```python
from build123d import *

# Parameters (mm, degrees)
SKETCH1_W           = 91.44
SKETCH1_H           = 91.44
BOSS_EXTRUDE1_DEPTH = 3.175
SKETCH2_R           = 38.1
BOSS_EXTRUDE2_DEPTH = 2.286
SKETCH3_R           = 1.143
BOSS_EXTRUDE3_DEPTH = 4.572
SKETCH4_R           = 2.667
CUT_EXTRUDE1_DEPTH  = 104.048504199
FILLET1_R           = 2.032
FILLET3_R           = 1.27
SKETCH5_R           = 20.32
CUT_EXTRUDE2_DEPTH  = 1.27
FILLET4_R           = 0.762
FILLET6_R           = 0.508


with BuildPart() as part:
    # Sketch1 → Boss-Extrude1 (new body)
    with BuildSketch(Plane(origin=(0, 0, 0), x_dir=(1, 0, 0), z_dir=(0, 1, 0))):
        with Locations((45.065298329, -2.727923628)):
            Rectangle(SKETCH1_W, SKETCH1_H)
    extrude(amount=BOSS_EXTRUDE1_DEPTH)

    # Sketch2 → Boss-Extrude2 (add)
    with BuildSketch(Plane(origin=(0, 3.175, 0), x_dir=(1, 0, 0), z_dir=(0, 1, 0))):
        with Locations(Location((45.065298329, -2.727923628, 0), (0, 0, 270))):
            Circle(SKETCH2_R)
    extrude(amount=BOSS_EXTRUDE2_DEPTH)

    # Sketch3 → Boss-Extrude3 (add)
    with BuildSketch(Plane(origin=(0, 3.175, 0), x_dir=(1, 0, 0), z_dir=(0, 1, 0))):
        with Locations(Location((4.425298329, 37.912076372, 0), (0, 0, 270))):
            Circle(SKETCH3_R)
        with Locations(Location((4.425298329, -43.367923628, 0), (0, 0, 270))):
            Circle(SKETCH3_R)
        with Locations(Location((85.705298329, -43.367923628, 0), (0, 0, 270))):
            Circle(SKETCH3_R)
        with Locations(Location((85.705298329, 37.912076372, 0), (0, 0, 270))):
            Circle(SKETCH3_R)
    extrude(amount=BOSS_EXTRUDE3_DEPTH)

    # Sketch4 → Cut-Extrude1 (cut, through all)
    with BuildSketch(Plane(origin=(0, 5.461, 0), x_dir=(1, 0, 0), z_dir=(0, 1, 0))):
        with Locations(Location((45.065298329, -2.727923628, 0), (0, 0, 270))):
            Circle(SKETCH4_R)
    extrude(amount=-CUT_EXTRUDE1_DEPTH, mode=Mode.SUBTRACT)

    # Fillet1
    fillet1_edges = [part.edges().sort_by_distance(p)[0] for p in [
        (45.065298329, 5.461, 0.060923628),
    ]]
    fillet(fillet1_edges, radius=FILLET1_R)

    # Fillet3
    fillet3_edges = [part.edges().sort_by_distance(p)[0] for p in [
        (-0.654701671, 1.5875, -42.992076372),
        (90.785298329, 1.5875, -42.992076372),
        (90.785298329, 1.5875, 48.447923628),
        (-0.654701671, 1.5875, 48.447923628),
    ]]
    fillet(fillet3_edges, radius=FILLET3_R)

    # Sketch5 → Cut-Extrude2 (cut)
    with BuildSketch(Plane.XZ):
        with Locations(Location((45.065298329, 2.727923628, 0), (0, 0, 270))):
            Circle(SKETCH5_R)
    extrude(amount=-CUT_EXTRUDE2_DEPTH, mode=Mode.SUBTRACT)

    # Fillet4
    fillet4_edges = [part.edges().sort_by_distance(p)[0] for p in [
        (45.065298329, 0, 23.047923628),
    ]]
    fillet(fillet4_edges, radius=FILLET4_R)

    # Fillet6
    fillet6_edges = [part.edges().sort_by_distance(p)[0] for p in [
        (45.065298329, 5.461, -35.372076372),
    ]]
    fillet(fillet6_edges, radius=FILLET6_R)


solid = part.part
```
Model file for the job. Use its own axes, mm. A direction names the side the tool comes from. Coordinates: 2 decimals unless noted, no trailing zeros. Answer as a JSON object with one key per item and string values.
Q1. Pull direction X, two halves, no side cores. Call faces 4 (the cylindrical face through (7.87, 4.05, -5.53)), 5 (the cylindrical face through (65.212, 1.012, 5.373)), 6 (the flat face through (86, 7.747, 43)): released by +X, released by -X, zero draft, split by the parting line, or undercut.
Report:
{"face 4": "split by the parting line", "face 5": "undercut", "face 6": "zero draft"}
Q2. Probe probe 1 along Y at (x, z) = (37.5, -28); probe 2 along Y at (x, z) = (27.5, 7.5); probe 3 along Z at (x, y) = (43.5, 1.75). List the from-to ranges inside material, lowest first.
Report:
{"probe 1": "y = 0 to 5.46", "probe 2": "y = 1.27 to 5.46", "probe 3": "z = -42.99 to 0.57, 4.89 to 48.45"}
Q3. 3-axis set-ups, long thin cutter, end or side, ignore diameter. For faces 1 (the cylindrical face through (86.84, 5.43, -38.06)), 2 (the flat face through (41, 1.27, 3)), 3 (the flat face through (90.785, 2, 3)): which of +Z, -Z, +X, -X, +Y, -Y reach the whole face in a straight line?
Report:
{"face 1": "+Y", "face 2": "-Y", "face 3": "+Z, -Z, +X, +Y, -Y"}
Q4. Flat gauge pins, fed straight in: P1, Ø6, axis at x = 45.07, z = 2.73, coming from the -Y side; P2, Ø3, axis at y = 6.5, z = -8.5, coming from the +X side; P3, Ø3, axis at x = 35.5, z = 16, coming from the +Y side. Where does each tip first touch, or does it go through?
Report:
{"P1": "stops at y = 1.27", "P2": "stops at x = 81.63", "P3": "stops at y = 5.46"}
